from build123d import *

# Parameters (mm, degrees)
PAD_DEPTH    = 50
SKETCH_W     = 10
SKETCH_H     = 54
PAD001_DEPTH = 80
SKETCH002_R  = 11
POCKET_DEPTH = 25.001


with BuildPart() as part:
    # Sketch001 → Pad (new body)
    with BuildSketch(Plane.XY):
        Polygon((-15, 0), (-15, 14.5), (-10, 12), (-10, 42), (-15, 39.5), (-15, 54), (-25, 54), (-25, 0), align=None)
    extrude(amount=PAD_DEPTH)

    # Sketch → Pad001 (join)
    with BuildSketch(Plane.XY):
        with Locations((-20, 27)):
            Rectangle(SKETCH_W, SKETCH_H)
    extrude(amount=PAD001_DEPTH)

    # Sketch002 → Pocket (cut, through all)
    with BuildSketch(Plane.YZ):
        with Locations((27, 65)):
            Circle(SKETCH002_R)
    extrude(amount=-POCKET_DEPTH, mode=Mode.SUBTRACT)


solid = part.part
The listing builds one solid part. Answer for the finished solid, in the listing's coordinates (mm). A direction names the side the tool comes from. Round coordinates to 2 decimals unless told otherwise and drop trailing zeros. Order: outer loops, then holes, each group sorted by start corner. A loop starts at its lowest first (then second) coordinate and runs counter-clockwise, first axis right, second up. Notation, with made-up numbers: (-15.5, 12.5) -> (6.5, 12.5) arc R15 cw to (6.5, 34.5) -> close; hole circle Ø6 at (89.25, 83). An arc over 180 degrees is marked (long way). Put each result on its own line as item: value.
Q1. Each of these flat-tipped pins is pushed along its axis until it touches: P1, Ø6, axis at x = -22.5, y = 45, coming from the -Z side; P2, Ø1.5, axis at x = -11.5, y = 20.5, coming from the +Z side. Where does it stop, or does it pass through?
Results list:
P1: z = 0
P2: z = 50
Q2. Section A-A, the plane y = 27 is taken. Write down the section's boundary in (x, z), and give its area (3 significant figures).
Results list:
outline: (-25, 0) -> (-10, 0) -> (-10, 50) -> (-15, 50) -> (-15, 54) -> (-25, 54) -> close; (-25, 76) -> (-15, 76) -> (-15, 80) -> (-25, 80) -> close
area: 830 mm^2
Q3. Which of the six approach directions +Z, -Z, +X, -X, +Y, -Y give full straight-line access (tool end or side, diameter ignored) to faces 1 (the flat face through (-13, 27, 50)), 2 (the flat face through (-20, 54, 39)), 3 (the flat face through (-12, 41, 25))?
Results list:
face 1: +Z, +X, +Y, -Y
face 2: +Z, -Z, +X, -X, +Y
face 3: +Z, -Z, +Y
Q4. Section D-D, the plane y = 41 is taken. Write down the section's boundary in (x, z).
Results list:
outline: (-25, 0) -> (-15, 0) -> (-15, 80) -> (-25, 80) -> close; (-12, 0) -> (-10, 0) -> (-10, 50) -> (-12, 50) -> close
Q5. Section B-B, the plane z = 65 is taken. Write down the section's boundary in (x, y).
Results list:
outline: (-25, 0) -> (-15, 0) -> (-15, 16) -> (-25, 16) -> close; (-25, 38) -> (-15, 38) -> (-15, 54) -> (-25, 54) -> close
Q6. Section C-C, the plane x = -19.25 is taken. Write down the section's boundary in (y, z), and give its area (3 significant figures).
Results list:
outline: (0, 0) -> (54, 0) -> (54, 80) -> (0, 80) -> close; hole circle Ø22 at (27, 65)
area: 3,940 mm^2
Q7. Determine the mould class of faces 4 (the flat face through (-19, 27, 0)), 5 (the flat face through (-12.54, 13.27, 24.65)), 6 (the flat face through (-10, 27, 25)) for opening direction X: pulls with the +X half, pulls with the -X half, needs draft (parallel to the pull), parting line crosses it, or undercut.
Results list:
face 4: needs draft
face 5: undercut
face 6: pulls with the +X half
Q8. Consider line 1 along Z through (x, y) = (-20.75, 27); line 2 along Y through (x, z) = (-19, 57); line 3 along Z through (x, y) = (-19.25, 34.5). Determine where each line is inside the solid, lowest interval first.
Results list:
line 1: 0 to 54, 76 to 80
line 2: 0 to 19.45, 34.55 to 54
line 3: 0 to 56.95, 73.05 to 80
